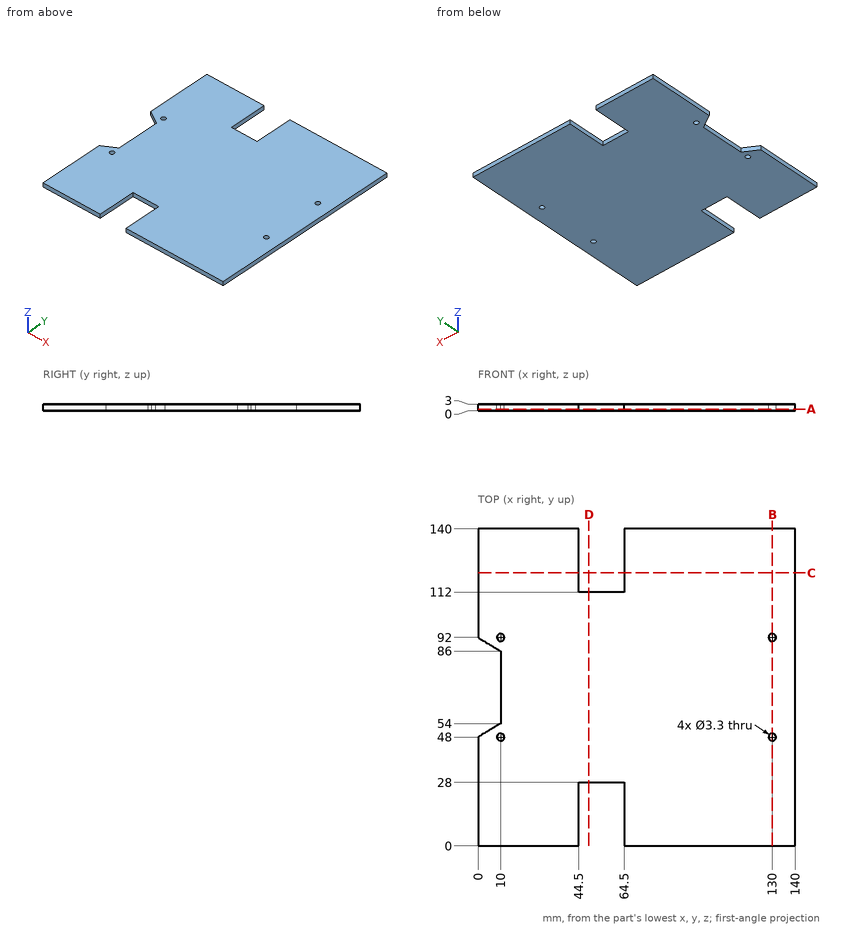
Can you work these out from the drawing? Everything is in mm from the part's minimum corner. Round coordinates to 2 decimals unless told otherwise and drop trailing zeros. Loops run counter-clockwise (first coordinate to the right, second up) from the corner with the lowest first, then second, coordinate; pieces in that order, holes last.
1. If we section it at C-C on y = 120.5: Write out the boundary of the cut face in (x, z), plus the area to 3 significant figures.
Answer list:
outline: (0, 0) - (44.5, 0) - (44.5, 3) - (0, 3) - close; (64.5, 0) - (140, 0) - (140, 3) - (64.5, 3) - close
area: 360 mm2
2. If we section it at A-A on z = 0.7: Write out the boundary of the cut face in (x, y).
Answer list:
outline: (0, 0) - (44.5, 0) - (44.5, 28) - (64.5, 28) - (64.5, 0) - (140, 0) - (140, 140) - (64.5, 140) - (64.5, 112) - (44.5, 112) - (44.5, 140) - (0, 140) - (0, 92) - (10, 86) - (10, 54) - (0, 48) - close; hole circle Ø3.3 at (10, 48); hole circle Ø3.3 at (10, 92); hole circle Ø3.3 at (130, 48); hole circle Ø3.3 at (130, 92)
3. For P1, Ø0.9, axis at x = 58.5, z = 1.5, coming from the +Y side; P2, Ø3, axis at x = 10, y = 92, coming from the +Z side; P3, Ø0.9, axis at y = 64, z = 1.5, coming from the -X side; P4, Ø6, axis at x = 73, y = 65.5, coming from the -Z side, each with a flat end and sliding along its axis, tell me the tip position at first contact or that it passes through.
Answer list:
P1: stops at y = 112
P2: passes through
P3: stops at x = 10
P4: stops at z = 0
4. If I drill on line 1 along X through (y, z) = (92, 2.4); line 2 along Y through (x, z) = (130, 2.3); line 3 along X through (y, z) = (124.5, 2.35), over which ranges is the centre line in solid material (lowest first)?
Answer list:
line 1: x = 0 to 8.35, 11.65 to 128.35, 131.65 to 140
line 2: y = 0 to 46.35, 49.65 to 90.35, 93.65 to 140
line 3: x = 0 to 44.5, 64.5 to 140
5. If we section it at D-D on x = 49: Write out the boundary of the cut face in (y, z).
Answer list:
outline: (28, 0) - (112, 0) - (112, 3) - (28, 3) - close
6. If we section it at B-B on x = 130: Write out the boundary of the cut face in (y, z).
Answer list:
outline: (0, 0) - (46.35, 0) - (46.35, 3) - (0, 3) - close; (49.65, 0) - (90.35, 0) - (90.35, 3) - (49.65, 3) - close; (93.65, 0) - (140, 0) - (140, 3) - (93.65, 3) - close
